For this review, take the finished solid that the model builds, in its own axes (mm). Round coordinates to 2 decimals unless told otherwise and drop trailing zeros. Loops run counter-clockwise (first coordinate to the right, second up) from the corner with the lowest first, then second, coordinate; pieces in that order, holes last. Notation, with made-up numbers: M 74,55 L 105,55 A25 ccw 105,81 Z; hole C 11.25,69.25 d3. An arc over 180 degrees is marked long. One line per question, with ' | ' between items. Start each with the question number.
1) We need section D-D (x = 40.5). Give the boundary of the cut face in (y, z).
2) We need section B-B (x = -12.5). Give the boundary of the cut face in (y, z).
3) We need section C-C (y = 0). Give the boundary of the cut face in (x, z), and give its area (3 significant figures).
4) Mouldability with a two-part tool opening along Y and no side actions: class faces 1 (the face through (87.5, -1, 5)), 2 (the face through (-1, -65, 5)), 3 (the face through (-64.13, 32.68, 4.93)), 4 (the face through (60.87, -47.32, 4.93)) as pulls with the +Y half, pulls with the -Y half, needs draft (parallel to the pull), parting line crosses it, or undercut.
5) For probe 1 along Y at (x, z) = (-62.5, 7.5); probe 2 along Y at (x, z) = (64.5, 3.25), list the stretches that pass through material, from the lowest coordinate up. Write a range as from..to.
6) We need section A-A (z = 6.25). State how many separate pieces and enclosed holes the cut face has, and give its area (3 significant figures).
```python
from build123d import *

# Parameters (mm, degrees)
F0_W     = 175
F0_H     = 130
F0_R     = 7.5
F1_DEPTH = 10


with BuildPart() as f1:
    # F0 (on Top) → F1 (new body)
    with BuildSketch(Plane.XY):
        Rectangle(F0_W, F0_H)
        with Locations((-62.5, -40)):
            Circle(F0_R, mode=Mode.SUBTRACT)
        with Locations((-37.5, -40)):
            Circle(F0_R, mode=Mode.SUBTRACT)
        with Locations((-12.5, -40)):
            Circle(F0_R, mode=Mode.SUBTRACT)
        with Locations((12.5, -40)):
            Circle(F0_R, mode=Mode.SUBTRACT)
        with Locations((37.5, -40)):
            Circle(F0_R, mode=Mode.SUBTRACT)
        with Locations((62.5, -40)):
            Circle(F0_R, mode=Mode.SUBTRACT)
        with Locations((-62.5, 0)):
            Circle(F0_R, mode=Mode.SUBTRACT)
        with Locations((-37.5, 0)):
            Circle(F0_R, mode=Mode.SUBTRACT)
        with Locations((-12.5, 0)):
            Circle(F0_R, mode=Mode.SUBTRACT)
        with Locations((-62.5, 40)):
            Circle(F0_R, mode=Mode.SUBTRACT)
        with Locations((-37.5, 40)):
            Circle(F0_R, mode=Mode.SUBTRACT)
        with Locations((-12.5, 40)):
            Circle(F0_R, mode=Mode.SUBTRACT)
        with Locations((12.5, 0)):
            Circle(F0_R, mode=Mode.SUBTRACT)
        with Locations((37.5, 0)):
            Circle(F0_R, mode=Mode.SUBTRACT)
        with Locations((62.5, 0)):
            Circle(F0_R, mode=Mode.SUBTRACT)
        with Locations((12.5, 40)):
            Circle(F0_R, mode=Mode.SUBTRACT)
        with Locations((37.5, 40)):
            Circle(F0_R, mode=Mode.SUBTRACT)
        with Locations((62.5, 40)):
            Circle(F0_R, mode=Mode.SUBTRACT)
    extrude(amount=F1_DEPTH)


solid = f1.part
```
Answers below:
1) outline: M -65,0 L -46.87,0 L -46.87,10 L -65,10 Z; M -33.13,0 L -6.87,0 L -6.87,10 L -33.13,10 Z; M 6.87,0 L 33.13,0 L 33.13,10 L 6.87,10 Z; M 46.87,0 L 65,0 L 65,10 L 46.87,10 Z
2) outline: M -65,0 L -47.5,0 L -47.5,10 L -65,10 Z; M -32.5,0 L -7.5,0 L -7.5,10 L -32.5,10 Z; M 7.5,0 L 32.5,0 L 32.5,10 L 7.5,10 Z; M 47.5,0 L 65,0 L 65,10 L 47.5,10 Z
3) outline: M -87.5,0 L -70,0 L -70,10 L -87.5,10 Z; M -55,0 L -45,0 L -45,10 L -55,10 Z; M -30,0 L -20,0 L -20,10 L -30,10 Z; M -5,0 L 5,0 L 5,10 L -5,10 Z; M 20,0 L 30,0 L 30,10 L 20,10 Z; M 45,0 L 55,0 L 55,10 L 45,10 Z; M 70,0 L 87.5,0 L 87.5,10 L 70,10 Z | area: 850 mm^2
4) face 1: needs draft | face 2: pulls with the -Y half | face 3: undercut | face 4: undercut
5) probe 1: -65..-47.5, -32.5..-7.5, 7.5..32.5, 47.5..65 | probe 2: -65..-47.23, -32.77..-7.23, 7.23..32.77, 47.23..65
6) separate pieces: 1 | enclosed holes: 18 | area: 19,600 mm^2
